```python
from build123d import *

# Parameters (mm, degrees)
SKETCH1_R           = 16.02
BOSS_EXTRUDE1_DEPTH = 0.38
SKETCH2_R           = 16.4
BOSS_EXTRUDE2_DEPTH = 11.94
SKETCH3_R           = 16.02
BOSS_EXTRUDE3_DEPTH = 0.38
SKETCH4_R           = 9.525
BOSS_EXTRUDE4_DEPTH = 12.32
SKETCH5_R           = 9.525
BOSS_EXTRUDE5_DEPTH = 0.38
BOSS_EXTRUDE5_TAPER = 45
SKETCH6_R           = 3.19
CUT_EXTRUDE1_DEPTH  = 19.05
SKETCH7_R           = 12.32
CUT_EXTRUDE5_DEPTH  = 0.38
CUT_EXTRUDE5_TAPER  = -45
SKETCH11_R          = 12.7
CUT_EXTRUDE6_DEPTH  = 5.97
SKETCH13_R          = 2.02
CUT_EXTRUDE7_DEPTH  = 10.97


with BuildPart() as part:
    # Sketch1 → Boss-Extrude1 (new body)
    with BuildSketch(Plane(origin=(0, 0, 0), x_dir=(1, 0, 0), z_dir=(0, 1, 0))):
        Circle(SKETCH1_R)
    extrude(amount=BOSS_EXTRUDE1_DEPTH)

    # Sketch2 → Boss-Extrude2 (add)
    with BuildSketch(Plane(origin=(0, 0.38, 0), x_dir=(1, 0, 0), z_dir=(0, 1, 0))):
        Circle(SKETCH2_R)
    extrude(amount=BOSS_EXTRUDE2_DEPTH)

    # Sketch3 → Boss-Extrude3 (add)
    with BuildSketch(Plane(origin=(0, 12.32, 0), x_dir=(1, 0, 0), z_dir=(0, 1, 0))):
        Circle(SKETCH3_R)
    extrude(amount=BOSS_EXTRUDE3_DEPTH)

    # Sketch4 → Boss-Extrude4 (add)
    with BuildSketch(Plane(origin=(0, 12.7, 0), x_dir=(1, 0, 0), z_dir=(0, 1, 0))):
        Circle(SKETCH4_R)
    extrude(amount=BOSS_EXTRUDE4_DEPTH)

    # Sketch5 → Boss-Extrude5 (add)
    with BuildSketch(Plane(origin=(0, 25.02, 0), x_dir=(1, 0, 0), z_dir=(0, 1, 0))):
        Circle(SKETCH5_R)
    extrude(amount=BOSS_EXTRUDE5_DEPTH, taper=BOSS_EXTRUDE5_TAPER)

    # Sketch6 → Cut-Extrude1 (cut)
    with BuildSketch(Plane(origin=(0, 25.4, 0), x_dir=(1, 0, 0), z_dir=(0, 1, 0))):
        Circle(SKETCH6_R)
    extrude(amount=-CUT_EXTRUDE1_DEPTH, mode=Mode.SUBTRACT)

    # Sketch7 → Cut-Extrude5 (cut)
    with BuildSketch(Plane(origin=(0, 6.35, 0), x_dir=(1, 0, 0), z_dir=(0, 1, 0))):
        Circle(SKETCH7_R)
    extrude(amount=-CUT_EXTRUDE5_DEPTH, taper=CUT_EXTRUDE5_TAPER, mode=Mode.SUBTRACT)

    # Sketch11 → Cut-Extrude6 (cut)
    with BuildSketch(Plane(origin=(0, 5.97, 0), x_dir=(1, 0, 0), z_dir=(0, 1, 0))):
        Circle(SKETCH11_R)
    extrude(amount=-CUT_EXTRUDE6_DEPTH, mode=Mode.SUBTRACT)

    # Sketch13 → Cut-Extrude7 (cut)
    with BuildSketch(Plane.XY):
        with Locations((0, 18.86)):
            Circle(SKETCH13_R)
    extrude(amount=-CUT_EXTRUDE7_DEPTH, mode=Mode.SUBTRACT)


solid = part.part
```
Design review of the part built by this model. Coordinates are the model's own, in mm. A direction names the side the tool comes from. Coordinates: 2 decimals unless noted, no trailing zeros. Write each loop counter-clockwise with the first axis right and the second up, starting at its lowest first coordinate (ties: lowest second). Pieces come first, ordered by that corner, then holes.
1) Add section A-A (x = 0). State how many separate pieces and enclosed holes the cut face has, plus the area to 3 significant figures.
2) Add section C-C (x = 13.5). Write out the cut boundary in (y, z), plus the area to 3 significant figures.
3) Add section B-B (y = 15). Write out the cut boundary in (x, z) (3 decimals), plus the area to 3 significant figures.
4) Insertion check: pin 1 (5 mm diameter, centred on x = 2.5, y = 22, fed in from -Z) (3 decimals); pin 2 (4 mm diameter, centred on x = 9, z = 10, fed in from +Y); pin 3 (7.5 mm diameter, centred on x = 0, z = 0, fed in from +Y); pin 4 (3 mm diameter, centred on x = -9, y = 4.5, fed in from +Z). Each pin has a flat end and moves straight along its axis. Give the tip position at first contact, or say it passes through.
5) Add section D-D (y = 18.86). Write out the cut boundary in (x, z) (3 decimals), plus the area to 3 significant figures.
6) Mouldability with a two-part tool opening along X and no side actions: class faces 6 (the flat face through (14.5, 0.38, 7.2)), 7 (the cylindrical face through (15.28, 12.51, -4.81)), 8 (the cylindrical face through (-0.692, 16.008, 3.114)) as +X half, -X half, draft (parallel to the pull), parting line (faces both ways), or undercut.
7) To check wall thickness, follow L1, parallel to Z at x = 0, y = 4.1; L2, parallel to X at y = 17.75, z = 0 (3 decimals). State the ranges of each line that lie inside material, in increasing order.
8) Machinability: for faces 1 (the flat face through (7, 12.7, 7)), 2 (the flat face through (-5, 0, -12)), 3 (the flat face through (4, 25.4, 0)), 4 (the cylindrical face through (-0.44, 16.89, -5.95)), 5 (the flat face through (3, 6.35, 3)), which of the approach directions +Z, -Z, +X, -X, +Y, -Y give a long, thin tool a straight path to every point of the face, cutting with its end or side? Answer none if there is none.
Check result:
1. separate pieces: 3
1. enclosed holes: 0
1. area: 349 mm2
2. outline: (0, -8.62) - (0.38, -8.62) - (0.38, -9.31) - (12.32, -9.31) - (12.32, -8.62) - (12.7, -8.62) - (12.7, 8.62) - (12.32, 8.62) - (12.32, 9.31) - (0.38, 9.31) - (0.38, 8.62) - (0, 8.62) - close
2. area: 235 mm2
3. outline: circle Ø19.05 at (0, 0); hole circle Ø6.38 at (0, 0)
3. area: 253 mm2
4. pin 1: stops at z = -9.525
4. pin 2: stops at y = 12.7
4. pin 3: stops at y = 25.4
4. pin 4: stops at z = 14.58
5. outline: (-2.02, -9.308) - (-2.02, -2.469) arc R3.19 cw (long way) to (2.02, -2.469) - (2.02, -9.308) arc R9.525 ccw (long way) to start
5. area: 227 mm2
6. face 6: draft
6. face 7: parting line
6. face 8: undercut
7. L1: z = -16.4 to -12.7, 12.7 to 16.4
7. L2: x = -9.525 to -3.19, 3.19 to 9.525
8. face 1: +Y
8. face 2: +Z, -Z, +X, -X, -Y
8. face 3: +Z, -Z, +X, -X, +Y
8. face 4: -Z
8. face 5: -Y
